For this review, use the dimensioned drawing (mm, ordinates from the lowest corner) and the shaded views. A direction names the side the tool comes from. Coordinates: 2 decimals unless noted, no trailing zeros. Loops run counter-clockwise (first coordinate to the right, second up) from the corner with the lowest first, then second, coordinate; pieces in that order, holes last. Notation, with made-up numbers: M -10.5,20.5 L 23.5,20.5 A11 cw 23.5,38.5 Z; hole C -20.75,85.25 d7. An arc over 180 degrees is marked long. One line per item, written item: value.
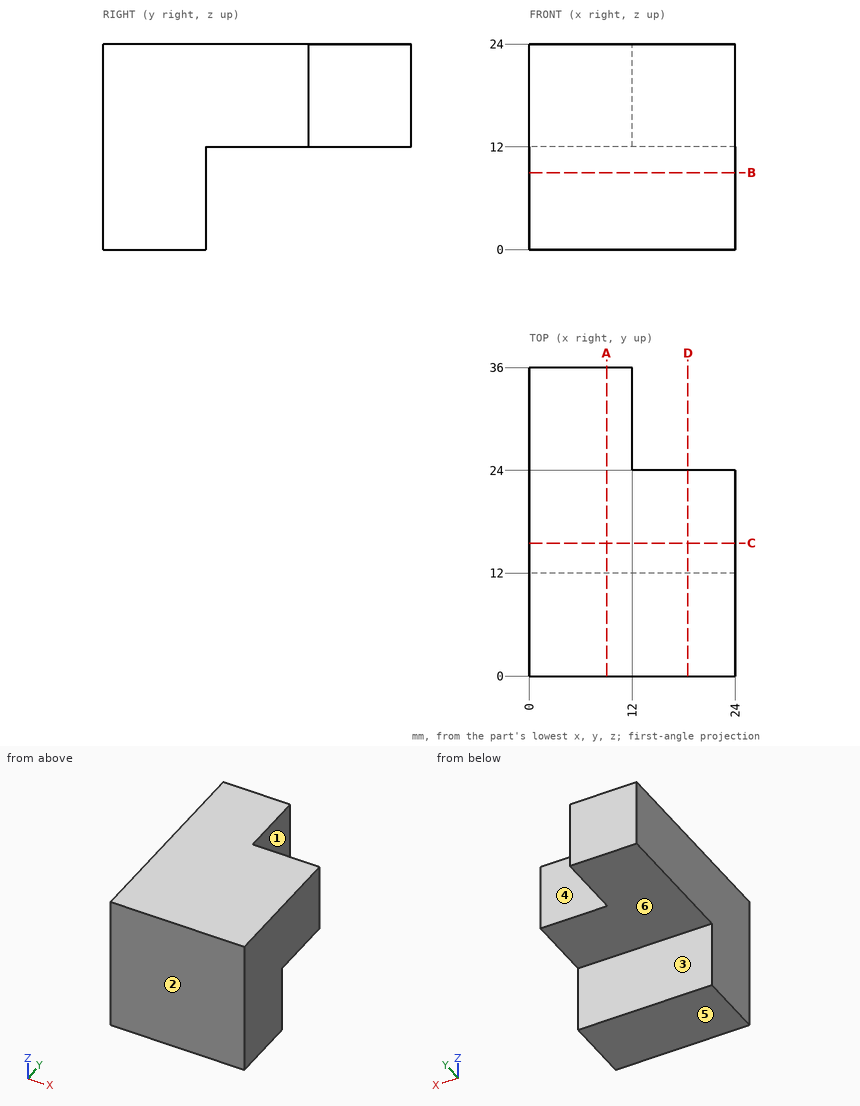
(1) Add section B-B on z = 9. State the section outline as (x, y) points.
Checks:
outline: M 0,0 L 24,0 L 24,12 L 0,12 Z
(2) Draft analysis for pull direction Y (two halves, no side actions). For the marked faces 1, 2 and 3, state which applies: pulls with the +Y half, pulls with the -Y half, needs draft (parallel to the pull), parting line crosses it, or undercut.
Checks:
face 1: needs draft
face 2: pulls with the -Y half
face 3: pulls with the +Y half
(3) Add section C-C on y = 15.5. State the section outline as (x, z) points, then the cut area to 3 significant figures.
Checks:
outline: M 0,12 L 24,12 L 24,24 L 0,24 Z
area: 288 mm^2
(4) Insertion check: pin 1 Ø2 at (x, z) = (6.5, 10) entering from +Y; pin 2 Ø12 at (x, y) = (8, 22.5) entering from -Z; pin 3 Ø3.5 at (x, z) = (20, 16) entering from +Y. Each pin has a flat end and moves straight along its axis. Give the tip position at first contact, or say it passes through.
Checks:
pin 1: y = 12
pin 2: z = 12
pin 3: y = 24
(5) Tool access review of the marked faces 4, 5 and 6: name each direction out of +Z, -Z, +X, -X, +Y, -Y from which nothing blocks a thin tool from reaching the whole face with its end or side.
Checks:
face 4: +Z, -Z, +X, +Y
face 5: -Z, +X, -X, +Y, -Y
face 6: -Z, +X, -X, +Y
(6) To check wall thickness, follow L1, parallel to Y at x = 22.5, z = 10.5; L2, parallel to Z at x = 19, y = 16.5. State the ranges of each line that lie inside material, in increasing order. Write a range as [from, to].
Checks:
L1: [0, 12]
L2: [12, 24]
(7) Add section A-A on x = 9. State the section outline as (y, z) points, then the cut area to 3 significant figures.
Checks:
outline: M 0,0 L 12,0 L 12,12 L 36,12 L 36,24 L 0,24 Z
area: 576 mm^2
(8) Add section D-D on x = 18.5. State the section outline as (y, z) points, then the cut area to 3 significant figures.
Checks:
outline: M 0,0 L 12,0 L 12,12 L 24,12 L 24,24 L 0,24 Z
area: 432 mm^2
